from build123d import *

# Parameters (mm, degrees)
EXTRUDE_1_DEPTH = 10
FILLET_1_R      = 4
EXTRUDE_2_DEPTH = 38


with BuildPart() as part:
    # 草圖1 → 填料-伸長1 (new body)
    with BuildSketch(Plane(origin=(0, 0, 0), x_dir=(0, 0, -1), z_dir=(1, 0, 0))):
        with BuildLine():
            Line((0, 0), (38, 0))
            Line((38, 0), (38, 36))
            Line((38, 36), (24.5, 36))
            Line((24.5, 36), (24.5, 25))
            ThreePointArc((24.5, 25), (19, 19.5), (13.5, 25))
            Line((13.5, 25), (13.5, 36))
            Line((13.5, 36), (0, 36))
            Line((0, 36), (0, 0))
        make_face()
    extrude(amount=EXTRUDE_1_DEPTH)

    # 圓角1
    fillet_1_edges = [part.edges().sort_by_distance(p)[0] for p in [
        (5, 36, 0),
        (5, 36, -38),
    ]]
    fillet(fillet_1_edges, radius=FILLET_1_R)

    # 草圖2 → 填料-伸長2 (add)
    with BuildSketch(Plane.XY):
        with BuildLine():
            Line((-64, 0), (-74, 0))
            ThreePointArc((-74, 0), (-51.08453427, 27.534478591), (-19.846606339, 10))
            Line((-19.846606339, 10), (0, 10))
            Line((0, 10), (0, 0))
            Line((0, 0), (-28, 0))
            ThreePointArc((-28, 0), (-46, 18), (-64, 0))
        make_face()
    extrude(amount=-EXTRUDE_2_DEPTH)


solid = part.part
Part model, mm, in its own coordinate system. A direction names the side the tool comes from. Round coordinates to 2 decimals unless told otherwise and drop trailing zeros. Order: outer loops, then holes, each group sorted by start corner. A loop starts at its lowest first (then second) coordinate and runs counter-clockwise, first axis right, second up. Notation, with made-up numbers: (-29, 75) -> (19, 75) arc R15 ccw to (19, 98) -> close; hole circle Ø2 at (-8.75, 62). An arc over 180 degrees is marked (long way). Put each result on its own line as item: value.
Q1. Tool access for faces 4 (the face through (5, 30, -13.5)), 5 (the face through (-10, 10, -19)), 6 (the face through (-46, 18, -19)): list every direction of +Z, -Z, +X, -X, +Y, -Y with a clear straight run to the whole face (end or side of a thin tool).
From the geometry:
face 4: +X, +Y
face 5: +Z, -Z, +Y
face 6: +Z, -Z, -Y
Q2. Band-saw the part on C-C (y = 24). Give the cut face in (x, z), and give its area (3 significant figures).
From the geometry:
outline: (-60.42, -38) -> (-31.58, -38) -> (-31.58, 0) -> (-60.42, 0) -> close; (0, -38) -> (10, -38) -> (10, -24.41) -> (0, -24.41) -> close; (0, -13.59) -> (10, -13.59) -> (10, 0) -> (0, 0) -> close
area: 1,370 mm2
Q3. Band-saw the part on D-D (x = -6). Give the cut face in (y, z), and give its area (3 significant figures).
From the geometry:
outline: (0, -38) -> (10, -38) -> (10, 0) -> (0, 0) -> close
area: 380 mm2
Q4. Pin check, flat tips, straight feed: pin 1 Ø13 at (y, z) = (28.5, -14.5) entering from -X; pin 2 Ø2 at (x, y) = (-53, 27) entering from +Z; pin 3 Ø4 at (x, z) = (-16.5, -30.5) entering from +Y; pin 4 Ø2 at (x, z) = (-33.5, -9) entering from -Y. Stop position of each tip, or through.
From the geometry:
pin 1: stops at x = -63.32
pin 2: stops at z = 0
pin 3: stops at y = 10
pin 4: stops at y = 11.91
Q5. Wall check: line 1 (X direction, y = 15.5, z = -19); line 2 (X direction, y = 16, z = -32.5); line 3 (X direction, y = 7, z = -1.5). Give the ranges that are in metal, low to high. Write a range as [from, to].
From the geometry:
line 1: x = [-69.32, -55.15], [-36.85, -22.68], [0, 10]
line 2: x = [-68.98, -54.25], [-37.75, -23.02], [0, 10]
line 3: x = [-73.11, -62.58], [-29.42, 10]
Q6. Band-saw the part on A-A (y = 30.5). Give the cut face in (x, z), and give its area (3 significant figures).
From the geometry:
outline: (0, -38) -> (10, -38) -> (10, -24.5) -> (0, -24.5) -> close; (0, -13.5) -> (10, -13.5) -> (10, 0) -> (0, 0) -> close
area: 270 mm2
Q7. Band-saw the part on B-B (z = -19). Give the cut face in (x, y).
From the geometry:
outline: (-74, 0) -> (-64, 0) arc R18 cw to (-28, 0) -> (10, 0) -> (10, 19.5) -> (0, 19.5) -> (0, 10) -> (-19.85, 10) arc R28 ccw to start
Q8. Pull direction Z, two halves, no side cores. Call faces 1 (the face through (4.9, 19.5, -19.1)), 2 (the face through (-31, 13, 0)), 3 (the face through (0, 17, -19)): pulls with the +Z half, pulls with the -Z half, needs draft (parallel to the pull), parting line crosses it, or undercut.
From the geometry:
face 1: undercut
face 2: pulls with the +Z half
face 3: needs draft
